Source: CAD feature listing. Evaluate the final solid. Frame: model axes, mm. A direction names the side the tool comes from. Coordinates: 2 decimals unless noted, no trailing zeros. Order: outer loops, then holes, each group sorted by start corner. A loop starts at its lowest first (then second) coordinate and runs counter-clockwise, first axis right, second up. Notation, with made-up numbers: (78.25, 76.5) -> (95.25, 76.5) arc R23 cw to (95.25, 95.5) -> close; hole circle Ø7 at (-27.75, 50.25). An arc over 180 degrees is marked (long way). Put each result on its own line as item: value.
from build123d import *

# Parameters (mm, degrees)
F2_DEPTH = 8
F3_DEPTH = 4
F4_DEPTH = 25


with BuildPart() as f2:
    # F0 (on Top) → F2 (new body)
    with BuildSketch(Plane.XY):
        with BuildLine():
            ThreePointArc((7.5, 0), (0, 7.5), (-7.5, 0))
            Line((-7.5, 0), (-2.5, 0))
            ThreePointArc((-2.5, 0), (0, 2.5), (2.5, 0))
            Line((2.5, 0), (7.5, 0))
        make_face()
    extrude(amount=F2_DEPTH)

    # F0 (on Top) → F3 (join)
    with BuildSketch(Plane.XY):
        with BuildLine():
            ThreePointArc((10, 0), (0, 10), (-10, 0))
            Line((-10, 0), (-7.5, 0))
            ThreePointArc((-7.5, 0), (0, 7.5), (7.5, 0))
            Line((7.5, 0), (10, 0))
        make_face()
        with BuildLine():
            ThreePointArc((7.5, 0), (0, 7.5), (-7.5, 0))
            Line((-7.5, 0), (-2.5, 0))
            ThreePointArc((-2.5, 0), (0, 2.5), (2.5, 0))
            Line((2.5, 0), (7.5, 0))
        make_face()
        with BuildLine():
            ThreePointArc((2.5, 0), (0, 2.5), (-2.5, 0))
            Line((-2.5, 0), (2.5, 0))
        make_face()
    extrude(amount=F3_DEPTH)

    # F4 (cut): a face of the model
    f4_faces = [f2.faces().sort_by_distance(p)[0] for p in [
        (0, 1.0610329539, 4),
    ]]
    extrude(f4_faces, amount=-F4_DEPTH, mode=Mode.SUBTRACT)


solid = f2.part
1. Pull-direction query (X, two-part tool) for faces 1 (the cylindrical face through (-0.1, 2.5, 3.9)), 2 (the cylindrical face through (0, 10, 2)), 3 (the flat face through (0, 4, 8)); classes: pulls with the +X half, pulls with the -X half, needs draft (parallel to the pull), parting line crosses it, or undercut.
Numbers:
face 1: undercut
face 2: parting line crosses it
face 3: needs draft
2. Cut plane D-D on z = 5.5. Output: boundary loops of the cut face in (x, y).
Numbers:
outline: (-7.5, 0) -> (-2.5, 0) arc R2.5 cw to (2.5, 0) -> (7.5, 0) arc R7.5 ccw to start
3. Set-up query: faces 4 (the flat face through (5, 0, 4)), 5 (the cylindrical face through (0.16, 7.5, 5.97)). Return all of +Z, -Z, +X, -X, +Y, -Y with unobstructed straight access to the full face (end or side cutting, diameter ignored); none if empty.
Numbers:
face 4: +Z, -Z, +X, -X, -Y
face 5: +Z, +Y
4. Cut plane A-A on y = 6. Output: boundary loops of the cut face in (x, z).
Numbers:
outline: (-8, 0) -> (8, 0) -> (8, 4) -> (4.5, 4) -> (4.5, 8) -> (-4.5, 8) -> (-4.5, 4) -> (-8, 4) -> close
5. Ray query, line 1 along Z through (x, y) = (8, 0.75); line 2 along X through (y, z) = (2, 4.75); line 3 along Y through (x, z) = (2.75, 3.75). Return the intervals inside material, ascending.
Numbers:
line 1: z = 0 to 4
line 2: x = -7.23 to -1.5, 1.5 to 7.23
line 3: y = 0 to 9.61
6. Cut plane B-B on y = 1.5. Output: boundary loops of the cut face in (x, z).
Numbers:
outline: (-9.89, 0) -> (-2, 0) -> (-2, 8) -> (-7.35, 8) -> (-7.35, 4) -> (-9.89, 4) -> close; (2, 0) -> (9.89, 0) -> (9.89, 4) -> (7.35, 4) -> (7.35, 8) -> (2, 8) -> close
7. First-contact query: pin 1 (1 mm diameter, centred on x = -2.5, y = 8, fed in from -Z). Flat tip, straight axial feed; report the tip coordinate or a pass-through.
Numbers:
pin 1: stops at z = 0
8. Cut plane C-C on x = 0. Output: boundary loops of the cut face in (y, z), plus the area to 3 significant figures.
Numbers:
outline: (2.5, 0) -> (10, 0) -> (10, 4) -> (7.5, 4) -> (7.5, 8) -> (2.5, 8) -> close
area: 50.0 mm2
